from build123d import *

# Parameters (mm, degrees)
SKETCH_W     = 110
SKETCH_H     = 36
PAD_DEPTH    = 3
SKETCH002_R  = 2
POCKET_DEPTH = 3
CHAMFER_SIZE = 1.99


with BuildPart() as part:
    # Sketch → Pad (new body)
    with BuildSketch(Plane.XY):
        Rectangle(SKETCH_W, SKETCH_H)
    extrude(amount=PAD_DEPTH)

    # Sketch002 (on Face6 of Pad) → Pocket (cut)
    with BuildSketch(Plane.XY.offset(3)):
        with Locations((-51, 14)):
            Circle(SKETCH002_R)
        with Locations((-51, -14)):
            Circle(SKETCH002_R)
        with Locations((51, -14)):
            Circle(SKETCH002_R)
        with Locations((51, 14)):
            Circle(SKETCH002_R)
    extrude(amount=-POCKET_DEPTH, mode=Mode.SUBTRACT)

    # Chamfer
    chamfer_edges = [part.edges().sort_by_distance(p)[0] for p in [
        (-53, 14, 3),
        (-53, -14, 3),
        (49, -14, 3),
        (49, 14, 3),
    ]]
    chamfer(chamfer_edges, length=CHAMFER_SIZE)


solid = part.part
Here's how the part is built. I have some questions about the finished solid (model axes, mm). Round coordinates to 2 decimals unless told otherwise and drop trailing zeros. Write each loop counter-clockwise with the first axis right and the second up, starting at its lowest first coordinate (ties: lowest second). Pieces come first, ordered by that corner, then holes.
1. Suppose I cut it at C-C (z = 2.2). List the corners of the cut face in (x, y) for me.
2. If we mould it in two halves opening along X, with no side actions, what happens to faces 1 (the cylindrical face through (49.526, -12.648, 0.512)), 2 (the flat face through (-55, 0, 1)), 3 (the flat face through (-1, 0, 3))? For each: released by +X, released by -X, zero draft, split by the parting line, or undercut.
3. I need wall thicknesses on L1, parallel to Y at x = -51, z = 0.55; L2, parallel to X at y = -15.5, z = 0.25. Which ranges of each line are inside material? Lowest first, please.
4. Suppose I cut it at A-A (x = -51). State how many separate pieces and enclosed holes the cut face has, and give its area (3 significant figures).
Answer sheet:
1. outline: (-55, -18) - (55, -18) - (55, 18) - (-55, 18) - close; hole circle Ø6.38 at (-51, -14); hole circle Ø6.38 at (-51, 14); hole circle Ø6.38 at (51, -14); hole circle Ø6.38 at (51, 14)
2. face 1: undercut
2. face 2: released by -X
2. face 3: zero draft
3. L1: y = -18 to -16, -12 to 12, 16 to 18
3. L2: x = -55 to -52.32, -49.68 to 49.68, 52.32 to 55
4. separate pieces: 3
4. enclosed holes: 0
4. area: 76.1 mm2
